Source: CAD feature listing. Evaluate the final solid. Frame: model axes, mm. Give positions to 0.01 mm unless a question says otherwise; leave off trailing zeros. Write each loop counter-clockwise with the first axis right and the second up, starting at its lowest first coordinate (ties: lowest second). Pieces come first, ordered by that corner, then holes. Notation, with made-up numbers: (-20, 2) -> (3, 2) arc R15 cw to (3, 19) -> close; hole circle Ø3 at (-20, 20.5). An arc over 180 degrees is marked (long way). Use one line per item in the form item = value. Start each with the question number.
(1) First-contact query: P1, Ø1.5, axis at x = 56, z = 0.5, coming from the +Y side. Flat tip, straight axial feed; report the tip coordinate or a pass-through.
(2) Cut plane B-B, the plane x = 0. Output: boundary loops of the cut face in (y, z), and give its area (3 significant figures).
(3) Cut plane D-D, the plane y = -13. Output: boundary loops of the cut face in (x, z), and give its area (3 significant figures).
(4) Cut plane C-C, the plane y = 0. Output: boundary loops of the cut face in (x, z), and give its area (3 significant figures).
(5) Material intervals for line 1 along X through (y, z) = (-23.5, 1.8); line 2 along Y through (x, z) = (45, 0.7); line 3 along Y through (x, z) = (0, 1.55), sorted ascending. Write a range as from..to.
(6) Cut plane A-A, the plane z = 2.05. Output: boundary loops of the cut face in (x, y), and give its area (3 significant figures).
from build123d import *

# Parameters (mm, degrees)
SKETCH_1_R      = 2.5
SKETCH_1_R_2    = 2
EXTRUDE_1_DEPTH = 3


with BuildPart() as part:
    # 草图1 → 凸台-拉伸1 (new body)
    with BuildSketch(Plane.XY):
        with BuildLine():
            Line((-55, -30.5), (0, -30.5))
            Line((0, -30.5), (55, -30.5))
            ThreePointArc((55, -30.5), (63.046888376, -28.809767542), (69.733665561, -24.024758746))
            Line((69.733665561, -24.024758746), (88.68341639, -3.381189686))
            ThreePointArc((88.68341639, -3.381189686), (88.803421515, 3.245610078), (82.240225301, 4.16936969))
            Line((82.240225301, 4.16936969), (58.798873493, -11.346848451))
            ThreePointArc((58.798873493, -11.346848451), (52.205164423, -14.439206454), (45, -15.5))
            Line((45, -15.5), (0, -15.5))
            Line((0, -15.5), (-45, -15.5))
            ThreePointArc((-45, -15.5), (-52.205164423, -14.439206454), (-58.798873493, -11.346848451))
            Line((-58.798873493, -11.346848451), (-82.240225301, 4.16936969))
            ThreePointArc((-82.240225301, 4.16936969), (-88.803421515, 3.245610078), (-88.68341639, -3.381189686))
            Line((-88.68341639, -3.381189686), (-69.733665561, -24.024758746))
            ThreePointArc((-69.733665561, -24.024758746), (-63.046888376, -28.809767542), (-55, -30.5))
        make_face()
        with Locations((85, 0)):
            Circle(SKETCH_1_R, mode=Mode.SUBTRACT)
        with Locations((-85, 0)):
            Circle(SKETCH_1_R, mode=Mode.SUBTRACT)
        with Locations((0, -23)):
            Circle(SKETCH_1_R, mode=Mode.SUBTRACT)
        with Locations((-45, -23)):
            Circle(SKETCH_1_R_2, mode=Mode.SUBTRACT)
        with Locations((45, -23)):
            Circle(SKETCH_1_R_2, mode=Mode.SUBTRACT)
    extrude(amount=EXTRUDE_1_DEPTH)


solid = part.part
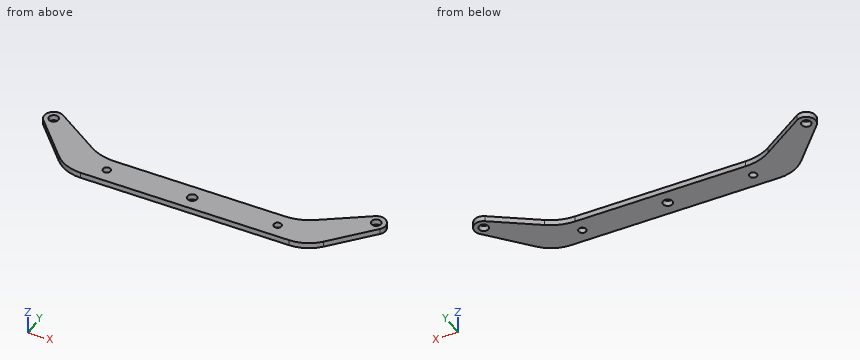
Geometry says:
q1.P1 = -12.57
q2.outline = (-30.5, 0) -> (-25.5, 0) -> (-25.5, 3) -> (-30.5, 3) -> close; (-20.5, 0) -> (-15.5, 0) -> (-15.5, 3) -> (-20.5, 3) -> close
q2.area = 30.0 mm^2
q3.outline = (-79.85, 0) -> (-55.9, 0) -> (-55.9, 3) -> (-79.85, 3) -> close; (55.9, 0) -> (79.85, 0) -> (79.85, 3) -> (55.9, 3) -> close
q3.area = 144 mm^2
q4.outline = (-90, 0) -> (-87.5, 0) -> (-87.5, 3) -> (-90, 3) -> close; (-82.5, 0) -> (-75.94, 0) -> (-75.94, 3) -> (-82.5, 3) -> close; (75.94, 0) -> (82.5, 0) -> (82.5, 3) -> (75.94, 3) -> close; (87.5, 0) -> (90, 0) -> (90, 3) -> (87.5, 3) -> close
q4.area = 54.4 mm^2
q5.line_1 = -70.22..-46.94, -43.06..-2.45, 2.45..43.06, 46.94..70.22
q5.line_2 = -30.5..-25, -21..-15.5
q5.line_3 = -30.5..-25.5, -20.5..-15.5
q6.outline = (-88.68, -3.38) -> (-69.73, -24.02) arc R20 ccw to (-55, -30.5) -> (55, -30.5) arc R20 ccw to (69.73, -24.02) -> (88.68, -3.38) arc R5 ccw to (82.24, 4.17) -> (58.8, -11.35) arc R25 cw to (45, -15.5) -> (-45, -15.5) arc R25 cw to (-58.8, -11.35) -> (-82.24, 4.17) arc R5 ccw to start; hole circle Ø5 at (-85, 0); hole circle Ø4 at (-45, -23); hole circle Ø5 at (0, -23); hole circle Ø4 at (45, -23); hole circle Ø5 at (85, 0)
q6.area = 2,750 mm^2
